Geometry check sheet. Reference: the model listing, model coordinates, mm. Face numbers are marked on the shaded views. A direction names the side the tool comes from. Coordinates: 2 decimals unless noted, no trailing zeros. Loops run counter-clockwise (first coordinate to the right, second up) from the corner with the lowest first, then second, coordinate; pieces in that order, holes last. Notation, with made-up numbers: M 67,55.5 L 111,55.5 A23 cw 111,65.5 Z; hole C 6.5,80.25 d5. An arc over 180 degrees is marked long. Use CSV: the item, a comma, the result in double quotes.
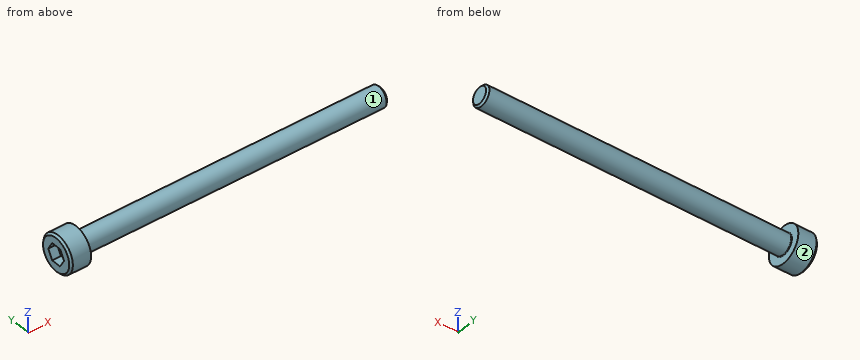
```python
from build123d import *

# Parameters (mm, degrees)
FILLET1_R   = 0.1
HEX_2_DEPTH = 1.3


with BuildPart() as part:
    # BodySke → Base-Revolve (revolve)
    with BuildSketch(Plane.XY):
        Polygon((0, 0), (0, 2.45), (0.3, 2.75), (3, 2.75), (3, 1.5), (47.7195, 1.5), (48, 1.2195), (48, 0), align=None)
    revolve(axis=Axis((-31.75, 0, 0), (1, 0, 0)))

    # Fillet1
    fillet1_edges = [part.edges().sort_by_distance(p)[0] for p in [
        (3, -1.5, 0),
    ]]
    fillet(fillet1_edges, radius=FILLET1_R)

    # Sketch2 → Hex-PreBroach (revolve, cut)
    with BuildSketch(Plane.XY):
        Polygon((0, 1.28), (1.3, 1.28), (2.039008345, 0), (0, 0), align=None)
    revolve(axis=Axis((0, 0, 0), (1, 0, 0)), mode=Mode.SUBTRACT)

    # Sketch3 → Hex 2 (cut)
    with BuildSketch(Plane(origin=(0, 0, 0), x_dir=(0, 0.5, 0.866025404), z_dir=(-1, 0, 0))):
        Polygon((0.739008345, 1.28), (-0.739008345, 1.28), (-1.478016689, 0), (-0.739008345, -1.28), (0.739008345, -1.28), (1.478016689, 0), align=None)
    extrude(amount=-HEX_2_DEPTH, mode=Mode.SUBTRACT)


solid = part.part
```
1. Set-up check for the marked faces 1 and 2: record each of +Z, -Z, +X, -X, +Y, -Y from which the full face is reachable in a straight line by a thin tool's end or side.
The answers:
face 1,"+X"
face 2,"+X, -X"
2. Gauge pin test, flat ends, axial feed: P1, Ø0.5, axis at y = -0.5, z = 1, coming from the -X side; P2, Ø0.6, axis at x = 0.5, y = -0.5, coming from the +Z side; P3, Ø3, axis at x = 24.5, z = -1.5, coming from the +Y side. Record the tip position at first contact, or that the pin passes through.
The answers:
P1,"x = 1.3"
P2,"z = 2.74"
P3,"y = 1.5"
3. Section check A-A, the plane x = 14.5. Record the cut outline in (y, z), plus the area to 3 significant figures.
The answers:
outline,"C 0,0 d3"
area,"7.07 mm^2"
4. Thickness scan on line 1 (X direction, y = 2, z = -0.9); line 2 (Z direction, x = 35, y = -0.15); line 3 (Z direction, x = 13, y = 1.3). Record the ranges inside material, lowest first. Write a range as [from, to].
The answers:
line 1,"[0, 3]"
line 2,"[-1.49, 1.49]"
line 3,"[-0.75, 0.75]"
